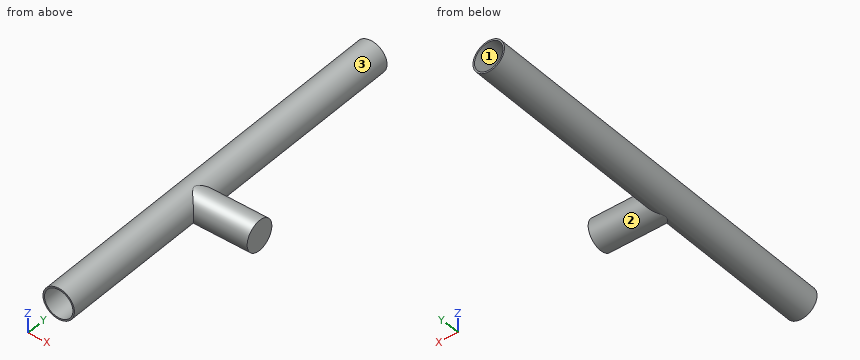
```python
from build123d import *

# Parameters (mm, degrees)
BOSS_EXTRUDE1_DEPTH      = 160
BOSS_EXTRUDE1_DEPTH_BACK = 5
SKETCH1_R                = 7.75
SKETCH1_R_2              = 7
SKETCH5_R                = 7.5
BOSS_EXTRUDE3_DEPTH      = 72.0622032
SKETCH7_R                = 7.75
SKETCH7_R_2              = 7
BOSS_EXTRUDE5_DEPTH      = 25
CUT_EXTRUDE1_START       = -38
SKETCH8_R                = 7.5
CUT_EXTRUDE1_DEPTH       = 38
SKETCH9_R                = 7
CUT_EXTRUDE2_DEPTH       = 105


with BuildPart() as part:
    # Sketch1 → Boss-Extrude1 (new, two sides: drawn at the far end of the back side and taken through both)
    with BuildSketch(Plane(origin=(0, 0, 0), x_dir=(1, 0, 0), z_dir=(0, 1, 0)).offset(-BOSS_EXTRUDE1_DEPTH_BACK)):
        with Locations(Location((0, 0, 0), (0, 0, 270))):
            Circle(SKETCH1_R)
        with Locations(Location((0, 0, 0), (0, 0, 270))):
            Circle(SKETCH1_R_2, mode=Mode.SUBTRACT)
    extrude(amount=BOSS_EXTRUDE1_DEPTH + BOSS_EXTRUDE1_DEPTH_BACK)

    # Sketch5 → Boss-Extrude3 (add)
    with BuildSketch(Plane(origin=(0, 0, 0), x_dir=(0, 0, -1), z_dir=(1, 0, 0))):
        with Locations(Location((0, 75, 0), (0, 0, 180))):
            Circle(SKETCH5_R)
    extrude(amount=BOSS_EXTRUDE3_DEPTH)

    # Sketch7 → Boss-Extrude5 (add)
    with BuildSketch(Plane(origin=(0, 160, 0), x_dir=(1, 0, 0), z_dir=(0, 1, 0))):
        with Locations(Location((0, 0, 0), (0, 0, 270))):
            Circle(SKETCH7_R)
        with Locations(Location((0, 0, 0), (0, 0, 270))):
            Circle(SKETCH7_R_2, mode=Mode.SUBTRACT)
    extrude(amount=BOSS_EXTRUDE5_DEPTH)

    # Sketch8 → Cut-Extrude1 (cut)
    with BuildSketch(Plane(origin=(72.0622032, 0, 0), x_dir=(0, 0, -1), z_dir=(1, 0, 0)).offset(CUT_EXTRUDE1_START)):
        with Locations(Location((0, 75, 0), (0, 0, 180))):
            Circle(SKETCH8_R)
    extrude(amount=CUT_EXTRUDE1_DEPTH, mode=Mode.SUBTRACT)

    # Sketch9 → Cut-Extrude2 (cut)
    with BuildSketch(Plane.XZ.offset(5)):
        with Locations(Location((0, 0, 0), (0, 0, 90))):
            Circle(SKETCH9_R)
    extrude(amount=-CUT_EXTRUDE2_DEPTH, mode=Mode.SUBTRACT)


solid = part.part
```
The model under review builds one solid part; all positions refer to its coordinate system, in mm. Face numbers are marked on the shaded views. Give positions to 0.01 mm unless a question says otherwise; leave off trailing zeros. Loops run counter-clockwise (first coordinate to the right, second up) from the corner with the lowest first, then second, coordinate; pieces in that order, holes last. Notation, with made-up numbers: (21, 71.25) - (80, 71.25) arc R12 ccw to (80, 79.25) - close; hole circle Ø11 at (-1.75, 80.5). An arc over 180 degrees is marked (long way). Answer as a JSON object with one key per item and string values.
Q1. Add section D-D on y = 10.5. State the section outline as (x, z) points, plus the area to 3 significant figures.
Worked out:
{"outline": "circle Ø15.5 at (0, 0); hole circle Ø14 at (0, 0)", "area": "34.8 mm^2"}
Q2. Insertion check: pin 1 (8 mm diameter, centred on x = 18.5, z = -2, fed in from +Y); pin 2 (6 mm diameter, centred on y = 110.5, z = -2, fed in from -X); pin 3 (5 mm diameter, centred on y = 146, z = -4.5, fed in from +X); pin 4 (4 mm diameter, centred on x = 2.5, y = 148, fed in from -Z). Each pin has a flat end and moves straight along its axis. Give the tip position at first contact, or say it passes through.
Worked out:
{"pin 1": "stops at y = 82.5", "pin 2": "stops at x = -7.75", "pin 3": "stops at x = 7.49", "pin 4": "stops at z = -7.73"}
Q3. To check wall thickness, follow line 1 along Z through (x, y) = (-0.5, 23); line 2 along X through (y, z) = (37, 0); line 3 along X through (y, z) = (73.5, 0). State the ranges of each line that lie inside material, in increasing order.
Worked out:
{"line 1": "z = -7.73 to -6.98, 6.98 to 7.73", "line 2": "x = -7.75 to -7, 7 to 7.75", "line 3": "x = -7.75 to -7, 7 to 34.06"}
Q4. Mouldability with a two-part tool opening along X and no side actions: class the marked faces 1, 2 and 3 as +X half, -X half, draft (parallel to the pull), parting line (faces both ways), or undercut.
Worked out:
{"face 1": "undercut", "face 2": "draft", "face 3": "parting line"}
Q5. Add section C-C on z = 0. State the section outline as (x, y) points, plus the area to 3 significant figures.
Worked out:
{"outline": "(-7.75, -5) - (-7, -5) - (-7, 185) - (-7.75, 185) - close; (7, -5) - (7.75, -5) - (7.75, 67.5) - (34.06, 67.5) - (34.06, 82.5) - (7.75, 82.5) - (7.75, 185) - (7, 185) - close", "area": "680 mm^2"}
Q6. Add section B-B on y = 75. State the section outline as (x, z) points, plus the area to 3 significant figures.
Worked out:
{"outline": "(1.95, -7.5) - (34.06, -7.5) - (34.06, 7.5) - (1.95, 7.5) arc R7.75 ccw (long way) to start; hole circle Ø14 at (0, 0)", "area": "452 mm^2"}
Q7. Add section A-A on x = 0. State the section outline as (y, z) points.
Worked out:
{"outline": "(-5, -7.75) - (185, -7.75) - (185, -7) - (-5, -7) - close; (-5, 7) - (185, 7) - (185, 7.75) - (-5, 7.75) - close"}
